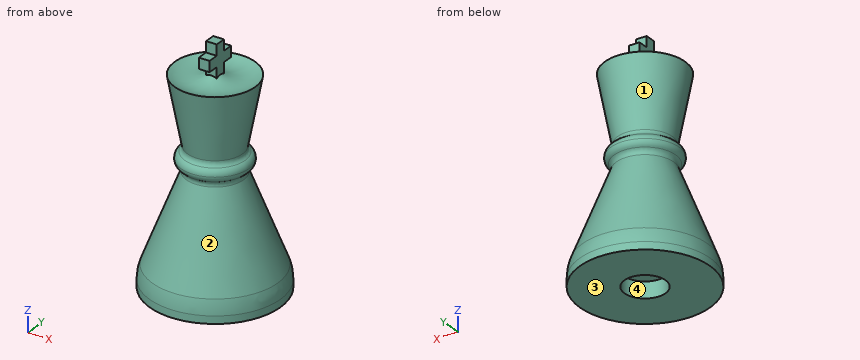
Autodesk Fusion 360 part; units mm, degrees
sketch "Esquisse1" plane through (0, 0, 0) normal (0, 1, 0) x (1, 0, 0)
  line L0 (0, 0) -> (13, 0)
  line L1 (13, 0) -> (0, 0)
  line L2 (0, 0) -> (0, -42)
  line L3 (13, 0) -> (13, -3)
  line L4 (8, -40) -> (5.3072, -25.7485)
  line L5 (13, -3) -> (5.3072, -22.8015)
  circle A0 centre (5.3072, -24.275) radius 1.4735
  line L6 (5.3072, -25.7485) -> (5.3072, -22.8015)
  line L7 (0, -42) -> (-0.7188, -42)
  arc A1 (8, -40) -> (-0.7188, -42) centre (4.75, -45.8363) ccw
  line L8 (0, 0) -> (4.1, 0)
  line L9 (4.1, 0) -> (4.1, -3.2)
  line L10 (4.1, -3.2) -> (0, -3.2)
  line L11 (0, -3.2) -> (0, 0)
  dimension "d1" = 13
  dimension "d2" = 42
  dimension "d3" = 3
  dimension "d4" = 4.1
  dimension "d5" = 3.2
revolve "Révolution1" add sketch "Esquisse1" angle 360 about axis through (0, 0, 0) along (0, 0, 1) contours L0 L1 L2 L3 L4 L5 A0 A1 L9 L10 | A0 L6 | A0 L6
fillet "Congé1" radius 1 2 edges at (-4.9481, -1.9192, 25.7485) (-4.9481, -1.9192, 22.8015)
fillet "Congé2" radius 8 1 edges at (-12.1203, -4.701, 3)
sketch "Esquisse2" plane through (0, 0, 0) normal (1, 0, 0) x (0, 1, 0)
  line L0 (-1.07, 40) -> (-1.07, 42.14)
  line L1 (-1.07, 42.14) -> (-3.21, 42.14)
  line L2 (-3.21, 42.14) -> (-3.21, 44.28)
  line L3 (-3.21, 44.28) -> (-1.07, 44.28)
  line L4 (-1.07, 44.28) -> (-1.07, 46.42)
  line L5 (-1.07, 46.42) -> (1.07, 46.42)
  line L6 (1.07, 46.42) -> (1.07, 44.28)
  line L7 (1.07, 44.28) -> (3.21, 44.28)
  line L8 (3.21, 44.28) -> (3.21, 42.14)
  line L9 (3.21, 42.14) -> (1.07, 42.14)
  line L10 (1.07, 42.14) -> (1.07, 40)
  line L11 (1.07, 40) -> (-1.07, 40)
  point P0 (0, 40)
  point P1 (0, 40)
  dimension "d12" = 2.14
extrude "Extrusion1" add sketch "Esquisse2" along normal blind 2.12 from surface at -1.06
Read the model definition and answer for the solid it produces. Units are mm, in the model's axes. Face numbers are marked on the shaded views. Coordinates: 2 decimals unless noted, no trailing zeros. Order: outer loops, then holes, each group sorted by start corner. A loop starts at its lowest first (then second) coordinate and runs counter-clockwise, first axis right, second up. Notation, with made-up numbers: (-7.75, -9) - (34.25, -9) arc R9 ccw to (34.25, -3) - close; hole circle Ø3 at (-2, 24.25). An arc over 180 degrees is marked (long way). Answer as a JSON object with one key per item and string values. Group by question number.
Item 1: The mould has two halves that part along Z. Classify the marked faces 1, 2, 3 and 4: +Z half, -Z half, draft (parallel to the pull), parting line (faces both ways), or undercut.
Item 2: Flat-ended cylindrical pins translate along their axes: P1, Ø12, axis at y = 1.5, z = 37.5, coming from the +X side; P2, Ø0.6, axis at x = 0.5, z = 43, coming from the +Y side; P3, Ø1.1, axis at x = 0, z = 45.5, coming from the +Y side. Find the tip coordinate at first contact, or state that the pin passes through.
Item 3: Section A-A (z = 36) is taken. Give the vertices of the cut face in (x, y), plus the area to 3 significant figures.
Item 4: Section B-B (z = 28) is taken. Give the vertices of the cut face in (x, y).
Item 5: Consider probe 1 along Y at (x, z) = (0, 1.6); probe 2 along Z at (x, y) = (10, 3); probe 3 along Z at (x, y) = (-10.5, 5.25). Determine where each line is inside the solid, lowest interval first. Write a range as from..to.
Results are:
{
 "1": {"face 1": "undercut", "face 2": "undercut", "face 3": "-Z half", "face 4": "draft"},
 "2": {"P1": "stops at x = 8", "P2": "stops at y = 3.21", "P3": "stops at y = 1.07"},
 "3": {"outline": "circle Ø14.49 at (0, 0)", "area": "165 mm^2"},
 "4": {"outline": "circle Ø11.47 at (0, 0)"},
 "5": {"probe 1": "y = -13..-4.1, 4.1..13", "probe 2": "z = 0..9.59", "probe 3": "z = 0..6.24"}
}
